Source: CAD feature listing. Evaluate the final solid. Frame: model axes, mm. A direction names the side the tool comes from. Round coordinates to 2 decimals unless told otherwise and drop trailing zeros. Loops run counter-clockwise (first coordinate to the right, second up) from the corner with the lowest first, then second, coordinate; pieces in that order, holes last. Notation, with made-up numbers: M 27,19.25 L 57,19.25 A27 cw 57,47.25 Z; hole C 6,65 d7. An arc over 180 degrees is marked long. One line per item, written item: value.
from build123d import *

# Parameters (mm, degrees)
RESSALTO_EXTRUS_O1_DEPTH = 87.5
ESBO_O2_R                = 8.5
CORTE_EXTRUS_O1_DEPTH    = 127.343539605


with BuildPart() as part:
    # Esboço1 → Ressalto-extrusão1 (new, symmetric)
    with BuildSketch(Plane(origin=(0, 0, 0), x_dir=(1, 0, 0), z_dir=(0, 1, 0))):
        with BuildLine():
            Line((-50, 0), (0, 0))
            Line((0, 0), (0, 76.2))
            Line((0, 76.2), (-2.35, 76.2))
            ThreePointArc((-2.35, 76.2), (-5.178427125, 75.028427125), (-6.35, 72.2))
            Line((-6.35, 72.2), (-6.35, 10.35))
            ThreePointArc((-6.35, 10.35), (-7.521572875, 7.521572875), (-10.35, 6.35))
            Line((-10.35, 6.35), (-50, 6.35))
            Line((-50, 6.35), (-50, 0))
        make_face()
    extrude(amount=RESSALTO_EXTRUS_O1_DEPTH, both=True)

    # Esboço2 → Corte-extrusão1 (cut, through all)
    with BuildSketch(Plane(origin=(0, 0, 0), x_dir=(0, 0, -1), z_dir=(1, 0, 0))):
        with Locations((41.27, 67.5)):
            Circle(ESBO_O2_R)
        with Locations((41.27, 33.75)):
            Circle(ESBO_O2_R)
        with Locations((41.27, 0)):
            Circle(ESBO_O2_R)
        with Locations((41.27, -33.75)):
            Circle(ESBO_O2_R)
        with Locations((41.27, -67.5)):
            Circle(ESBO_O2_R)
        Polygon((61.2, 87.5), (76.2, 87.5), (76.2, 72.5), align=None)
        Polygon((76.2, -72.5), (76.2, -87.5), (61.2, -87.5), align=None)
    extrude(amount=-CORTE_EXTRUS_O1_DEPTH, mode=Mode.SUBTRACT)


solid = part.part
1. Ray query, line 1 (Y direction, x = -4.5, z = -41.27); line 2 (Y direction, x = -3.5, z = -35); line 3 (Z direction, x = -11.5, y = -43). Return the intervals inside material, ascending. Write a range as [from, to].
Report:
line 1: y = [-87.5, -76], [-59, -42.25], [-25.25, -8.5], [8.5, 25.25], [42.25, 59], [76, 87.5]
line 2: y = [-87.5, -73.24], [-61.76, -39.49], [-28.01, -5.74], [5.74, 28.01], [39.49, 61.76], [73.24, 87.5]
line 3: z = [-6.35, 0]
2. Pin query (flat end, axial travel): pin 1 (10 mm diameter, centred on x = -22.5, y = 67, fed in from +Z); pin 2 (18.5 mm diameter, centred on y = 31.5, z = -41, fed in from -X); pin 3 (12 mm diameter, centred on x = -24, y = -6, fed in from -Z). Return the tip coordinate at first contact, or that it passes through.
Report:
pin 1: stops at z = 0
pin 2: stops at x = -6.35
pin 3: stops at z = -6.35
3. Section query C-C (z = -63). Return the cut outline in (x, y).
Report:
outline: M -6.35,-85.7 L 0,-85.7 L 0,85.7 L -6.35,85.7 Z
4. Section query B-B (z = -41.27). Return the cut outline in (x, y), and give its area (4 significant figures).
Report:
outline: M -6.35,-87.5 L 0,-87.5 L 0,-76 L -6.35,-76 Z; M -6.35,-59 L 0,-59 L 0,-42.25 L -6.35,-42.25 Z; M -6.35,-25.25 L 0,-25.25 L 0,-8.5 L -6.35,-8.5 Z; M -6.35,8.5 L 0,8.5 L 0,25.25 L -6.35,25.25 Z; M -6.35,42.25 L 0,42.25 L 0,59 L -6.35,59 Z; M -6.35,76 L 0,76 L 0,87.5 L -6.35,87.5 Z
area: 571.5 mm2
5. Section query D-D (x = -28). Return the cut outline in (y, z), and give its area (3 significant figures).
Report:
outline: M -87.5,-6.35 L 87.5,-6.35 L 87.5,0 L -87.5,0 Z
area: 1,110 mm2
6. Reachability of faces 4 (the face through (-30, 1, -6.35)), 5 (the face through (-5, 87.5, -17)) from +Z, -Z, +X, -X, +Y, -Y: full face, straight path, thin tool, end or side. Return the list, or none.
Report:
face 4: -Z, -X, +Y, -Y
face 5: +Z, -Z, +X, -X, +Y
7. Pull-direction query (Z, two-part tool) for faces 1 (the face through (-3.1, 79.9, -68.8)), 2 (the face through (-50, 1, -3)), 3 (the face through (-3.13, 70.05, -49.38)); classes: released by +Z, released by -Z, zero draft, split by the parting line, or undercut.
Report:
face 1: released by -Z
face 2: zero draft
face 3: undercut
8. Section query A-A (y = 33.75). Return the cut outline in (x, z), and give its area (3 significant figures).
Report:
outline: M -50,-6.35 L -10.35,-6.35 A4 cw -6.35,-10.35 L -6.35,-32.77 L 0,-32.77 L 0,0 L -50,0 Z; M -6.35,-72.2 A4 ccw -2.35,-76.2 L 0,-76.2 L 0,-49.77 L -6.35,-49.77 Z
area: 653 mm2
